The listing builds one solid part. Answer for the finished solid, in the listing's coordinates (mm). A direction names the side the tool comes from. Give positions to 0.01 mm unless a question says otherwise; leave off trailing zeros. Write each loop counter-clockwise with the first axis right and the second up, starting at its lowest first coordinate (ties: lowest second). Pieces come first, ordered by that corner, then holes.
```python
from build123d import *

# Parameters (mm, degrees)
BOSS_EXTRUDE1_DEPTH = 6.35
SKETCH2_W           = 23.222409447
SKETCH2_H           = 25.4
BOSS_EXTRUDE2_DEPTH = 12.7
FILLET1_R           = 38.1
FILLET2_R           = 76.2
SKETCH3_R           = 3.175
CUT_EXTRUDE1_DEPTH  = 12.7
CIRPATTERN1_COUNT   = 4
SKETCH4_R           = 1.5875
SKETCH4_R_2         = 3.175
CUT_EXTRUDE2_DEPTH  = 212.417812192
SKETCH5_R           = 3.175
CUT_EXTRUDE3_DEPTH  = 212.417812192


with BuildPart() as part:
    # Sketch1 → Boss-Extrude1 (new body)
    with BuildSketch(Plane(origin=(0, 0, 0), x_dir=(0, 0, -1), z_dir=(1, 0, 0))):
        with BuildLine():
            Line((-25.4, 25.4), (0, 25.4))
            Line((0, 25.4), (25.4, 25.4))
            Line((25.4, 25.4), (25.4, 147.047409447))
            ThreePointArc((25.4, 147.047409447), (0, 149.225), (-25.4, 147.047409447))
            Line((-25.4, 147.047409447), (-25.4, 25.4))
        make_face()
        with BuildLine():
            Line((25.4, 25.4), (25.4, 0))
            Line((25.4, 0), (25.4, -25.4))
            Line((25.4, -25.4), (147.047409447, -25.4))
            ThreePointArc((147.047409447, -25.4), (148.679605696, -12.746586804), (149.225, 0))
            ThreePointArc((149.225, 0), (148.679605696, 12.746586804), (147.047409447, 25.4))
            Line((147.047409447, 25.4), (25.4, 25.4))
        make_face()
        with BuildLine():
            Line((-25.4, -25.4), (-25.4, 0))
            Line((-25.4, 0), (-25.4, 25.4))
            Line((-25.4, 25.4), (-147.047409447, 25.4))
            ThreePointArc((-147.047409447, 25.4), (-149.225, 0), (-147.047409447, -25.4))
            Line((-147.047409447, -25.4), (-25.4, -25.4))
        make_face()
        with BuildLine():
            Line((0, -149.225), (0, -25.4))
            Line((0, -25.4), (-25.4, -25.4))
            Line((-25.4, -25.4), (-25.4, -147.047409447))
            ThreePointArc((-25.4, -147.047409447), (-12.746586804, -148.679605696), (0, -149.225))
        make_face()
        with BuildLine():
            Line((25.4, -25.4), (0, -25.4))
            Line((0, -25.4), (0, -149.225))
            ThreePointArc((0, -149.225), (12.746586804, -148.679605696), (25.4, -147.047409447))
            Line((25.4, -147.047409447), (25.4, -25.4))
        make_face()
        with BuildLine():
            ThreePointArc((7.9502, 0), (5.621640332, -5.621640332), (0, -7.9502))
            Line((0, -7.9502), (0, -25.4))
            Line((0, -25.4), (25.4, -25.4))
            Line((25.4, -25.4), (25.4, 0))
            Line((25.4, 0), (7.9502, 0))
        make_face()
        with BuildLine():
            Line((0, -25.4), (0, -7.9502))
            ThreePointArc((0, -7.9502), (-5.621640332, -5.621640332), (-7.9502, 0))
            Line((-7.9502, 0), (-25.4, 0))
            Line((-25.4, 0), (-25.4, -25.4))
            Line((-25.4, -25.4), (0, -25.4))
        make_face()
        with BuildLine():
            Line((-25.4, 0), (-7.9502, 0))
            ThreePointArc((-7.9502, 0), (-5.621640332, 5.621640332), (0, 7.9502))
            Line((0, 7.9502), (0, 25.4))
            Line((0, 25.4), (-25.4, 25.4))
            Line((-25.4, 25.4), (-25.4, 0))
        make_face()
        with BuildLine():
            ThreePointArc((0, 7.9502), (5.621640332, 5.621640332), (7.9502, 0))
            Line((7.9502, 0), (25.4, 0))
            Line((25.4, 0), (25.4, 25.4))
            Line((25.4, 25.4), (0, 25.4))
            Line((0, 25.4), (0, 7.9502))
        make_face()
    extrude(amount=BOSS_EXTRUDE1_DEPTH)

    # Sketch2 → Boss-Extrude2 (add)
    with BuildSketch(Plane.ZY):
        with BuildLine():
            Line((-25.4, 147.047409447), (-25.4, 123.825))
            Line((-25.4, 123.825), (0, 123.825))
            Line((0, 123.825), (25.4, 123.825))
            Line((25.4, 123.825), (25.4, 147.047409447))
            ThreePointArc((25.4, 147.047409447), (0, 149.225), (-25.4, 147.047409447))
        make_face()
        with BuildLine():
            Line((147.047409447, 25.4), (123.825, 25.4))
            Line((123.825, 25.4), (123.825, 0))
            Line((123.825, 0), (123.825, -25.4))
            Line((123.825, -25.4), (147.047409447, -25.4))
            ThreePointArc((147.047409447, -25.4), (149.225, 0), (147.047409447, 25.4))
        make_face()
        with BuildLine():
            Line((0, -123.825), (-25.4, -123.825))
            Line((-25.4, -123.825), (-25.4, -147.047409447))
            ThreePointArc((-25.4, -147.047409447), (0, -149.225), (25.4, -147.047409447))
            Line((25.4, -147.047409447), (25.4, -123.825))
            Line((25.4, -123.825), (0, -123.825))
        make_face()
        with Locations((-135.436204723, -12.7)):
            Rectangle(SKETCH2_W, SKETCH2_H)
        with BuildLine():
            Line((-147.047409447, 0), (-147.047409447, 25.4))
            ThreePointArc((-147.047409447, 25.4), (-148.679605696, 12.746586804), (-149.225, 0))
            Line((-149.225, 0), (-147.047409447, 0))
        make_face()
        with BuildLine():
            Line((-147.047409447, -25.4), (-147.047409447, 0))
            Line((-147.047409447, 0), (-149.225, 0))
            ThreePointArc((-149.225, 0), (-148.679605696, -12.746586804), (-147.047409447, -25.4))
        make_face()
        with Locations((-135.436204723, 12.7)):
            Rectangle(SKETCH2_W, SKETCH2_H)
        with BuildLine():
            Line((-147.047409447, 0), (-147.047409447, 25.4))
            ThreePointArc((-147.047409447, 25.4), (-148.679605696, 12.746586804), (-149.225, 0))
            Line((-149.225, 0), (-147.047409447, 0))
        make_face()
        with BuildLine():
            Line((-147.047409447, -25.4), (-147.047409447, 0))
            Line((-147.047409447, 0), (-149.225, 0))
            ThreePointArc((-149.225, 0), (-148.679605696, -12.746586804), (-147.047409447, -25.4))
        make_face()
    extrude(amount=-BOSS_EXTRUDE2_DEPTH)

    # Fillet1
    fillet1_edges = [part.edges().sort_by_distance(p)[0] for p in [
        (3.175, -25.4, 25.4),
        (3.175, 25.4, 25.4),
        (3.175, 25.4, -25.4),
        (3.175, -25.4, -25.4),
    ]]
    fillet(fillet1_edges, radius=FILLET1_R)

    # Fillet2
    # the kernel refuses this fillet: 76.2 mm, written as the material it adds along each edge
    with BuildSketch(Plane(origin=(6.35, -25.4, 123.825), x_dir=(0, 0, -1), z_dir=(0, 1, 0)), Plane(origin=(6.35, -123.825, -25.4), x_dir=(0, 1, 0), z_dir=(0, 0, 1)), Plane(origin=(6.35, 25.4, -123.825), x_dir=(0, 0, 1), z_dir=(0, -1, 0)), Plane(origin=(6.35, 123.825, 25.4), x_dir=(0, -1, 0), z_dir=(0, 0, -1))) as fillet2_piece_1:
        with BuildLine():
            CenterArc((30.453530173, -76.2), FILLET2_R, 90, 23.556464309)
            Line((0, -6.35), (-0.609070603, -4.953))
            ThreePointArc((-0.609070603, -4.953), (-1.524, -3.175), (-1.524, 0))
            Line((-1.524, 0), (0, 1.524))
            Line((0, 1.524), (30.453530173, 1.524))
            Line((30.453530173, 1.524), (30.453530173, 0))
        make_face()
    extrude(amount=50.8)

    # Sketch3 → Cut-Extrude1 (cut)
    with BuildSketch(Plane(origin=(0, 0, -149.225), x_dir=(-1, 0, 0), z_dir=(0, 0, -1))):
        with Locations((-6.35, 12.7)):
            Circle(SKETCH3_R)
        with Locations((-6.35, -11.43)):
            Circle(SKETCH3_R)
    cut_extrude1 = extrude(amount=-CUT_EXTRUDE1_DEPTH, mode=Mode.SUBTRACT)

    # CirPattern1: Cut-Extrude1 ×4 about axis
    cirpattern1_axis = Axis((0, 0, 0), (1, 0, 0))
    for i in range(1, CIRPATTERN1_COUNT):
        add(cut_extrude1.rotate(cirpattern1_axis, i * 360 / CIRPATTERN1_COUNT), mode=Mode.SUBTRACT)

    # Sketch4 → Cut-Extrude2 (cut, through all)
    with BuildSketch(Plane.ZY):
        with Locations((73.9775, -12.7635)):
            Circle(SKETCH4_R)
        with Locations((54.9275, -12.7635)):
            Circle(SKETCH4_R)
        with Locations((19.05, 107.95)):
            Circle(SKETCH4_R_2)
        with Locations((-19.05, 107.95)):
            Circle(SKETCH4_R_2)
    extrude(amount=-CUT_EXTRUDE2_DEPTH, mode=Mode.SUBTRACT)

    # Sketch5 → Cut-Extrude3 (cut, through all)
    with BuildSketch(Plane.ZY):
        with Locations((2.163404924, -64.900779229)):
            Circle(SKETCH5_R)
        with Locations((-72.013510637, 9.276136331)):
            Circle(SKETCH5_R)
    extrude(amount=-CUT_EXTRUDE3_DEPTH, mode=Mode.SUBTRACT)


solid = part.part
```
Item 1: A cutting plane is placed at A-A, the plane y = 129. Give the vertices of the cut face in (x, z), plus the area to 3 significant figures.
Conclusion:
outline: (0, -25.4) - (12.7, -25.4) - (12.7, 25.4) - (0, 25.4) - close
area: 645 mm2
Item 2: Consider probe 1 along Z at (x, y) = (3.75, 107.95) (3 decimals); probe 2 along Y at (x, z) = (5, 89); probe 3 along Y at (x, z) = (4.25, -12.5) (3 decimals). Determine where each line is inside the solid, lowest interval first.
Conclusion:
probe 1: z = -25.4 to -22.225, -15.875 to 15.875, 22.225 to 25.4
probe 2: y = -25.4 to 25.4
probe 3: y = -136.525 to 136.525
Item 3: Determine the mould class of faces 1 (the face through (12.7, 0, -137)), 2 (the face through (5, -114, 25.4)), 3 (the face through (6, -11, -136.525)), 4 (the face through (6, 136.525, 13)) for opening direction Z: pulls with the +Z half, pulls with the -Z half, needs draft (parallel to the pull), parting line crosses it, or undercut.
Conclusion:
face 1: needs draft
face 2: pulls with the +Z half
face 3: pulls with the -Z half
face 4: undercut
Item 4: Which of the six approach directions +Z, -Z, +X, -X, +Y, -Y give full straight-line access (tool end or side, diameter ignored) to faces 5 (the face through (6.35, 22, 1)), 6 (the face through (6.76, 142.81, 15.85)), 7 (the face through (3.32, -142.85, 10.48)), 8 (the face through (5, 25.4, 114))?
Conclusion:
face 5: +X
face 6: +Y
face 7: -Y
face 8: +Z, +X, -X, +Y
Item 5: A cutting plane is placed at B-B, the plane z = -98.5. Give the vertices of the cut face in (x, y).
Conclusion:
outline: (0, -25.4) - (6.52, -25.4) - (6.52, 25.4) - (0, 25.4) - close
Item 6: Each of these flat-tipped pins is pushed along its axis until it touches: P1, Ø5.5, axis at x = 6.35, z = 11.43, coming from the -Y side (3 decimals); P2, Ø1.9, axis at x = 5.5, y = 10.5, coming from the +Z side (3 decimals); P3, Ø4, axis at x = 6, y = -97, coming from the +Z side; P4, Ø2.5, axis at y = -12.76, z = 73.98, coming from the -X side. Where does it stop, or does it pass through?
Conclusion:
P1: stops at y = -136.525
P2: stops at z = 136.525
P3: stops at z = 25.4
P4: passes through
